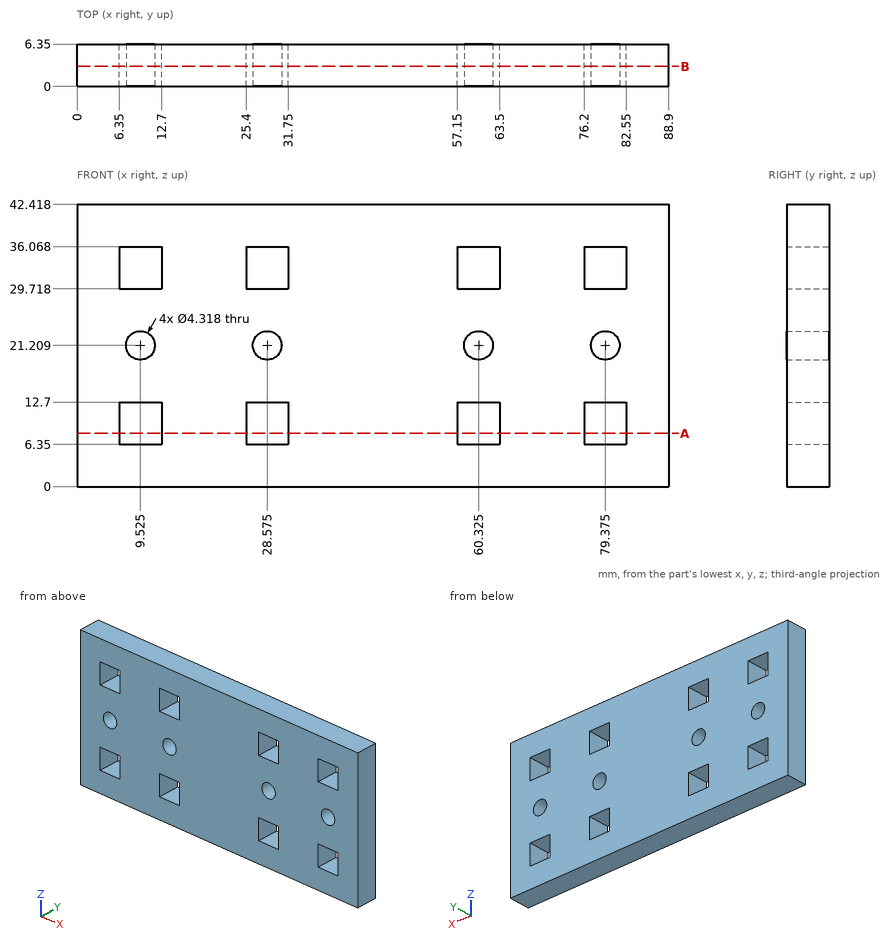
Can you work these out from the drawing? Everything is in mm from the part's minimum corner. Give positions to 0.01 mm unless a question says otherwise; leave off trailing zeros. Write each loop counter-clockwise with the first axis right and the second up, starting at its lowest first coordinate (ties: lowest second). Pieces come first, ordered by that corner, then holes. Notation, with made-up numbers: M 64,0.5 L 74,0.5 A27 ccw 74,21.5 Z; hole C 66.25,-12 d3. An arc over 180 degrees is marked long. Answer in a Markdown table with one row per item. Add a question column.
Item 1: Please list where these lines run through material, in increasing order: L1, parallel to X at y = 3.5, z = 12; L2, parallel to Z at x = 79.5, y = 5.75; L3, parallel to Z at x = 59.5, y = 5.
Item 2: Imagine slicing it at A-A, the plane z = 8. Write out the boundary of the cut face in (x, y).
Item 3: Imagine slicing it at B-B, the plane y = 3. State how many separate pieces and enclosed holes the cut face has, plus the area to 3 significant figures.
Evaluation:
| question | item | result |
|---|---|---|
| 1 | L1 | x = 0 to 6.35, 12.7 to 25.4, 31.75 to 57.15, 63.5 to 76.2, 82.55 to 88.9 |
| 1 | L2 | z = 0 to 6.35, 12.7 to 19.05, 23.36 to 29.72, 36.07 to 42.42 |
| 1 | L3 | z = 0 to 6.35, 12.7 to 19.21, 23.2 to 29.72, 36.07 to 42.42 |
| 2 | outline | M 0,0 L 6.35,0 L 6.35,6.35 L 0,6.35 Z; M 12.7,0 L 25.4,0 L 25.4,6.35 L 12.7,6.35 Z; M 31.75,0 L 57.15,0 L 57.15,6.35 L 31.75,6.35 Z; M 63.5,0 L 76.2,0 L 76.2,6.35 L 63.5,6.35 Z; M 82.55,0 L 88.9,0 L 88.9,6.35 L 82.55,6.35 Z |
| 3 | separate pieces | 1 |
| 3 | enclosed holes | 12 |
| 3 | area | 3,390 mm² |
